Part print with two shaded views. Sizes in mm from the minimum x, y, z corner. Round coordinates to 2 decimals unless told otherwise and drop trailing zeros. Loops run counter-clockwise (first coordinate to the right, second up) from the corner with the lowest first, then second, coordinate; pieces in that order, holes last. Notation, with made-up numbers: M -6,-30.5 L 52,-30.5 A23 cw 52,-1.5 Z; hole C 66.25,11 d6. An arc over 180 degrees is marked long. Use a Markdown table: item, result. Add a question column.
Item 1: Wall check: L1, parallel to Z at x = 31, y = 95; L2, parallel to Y at x = 50, z = 13.25; L3, parallel to Z at x = 79, y = 85. Give the ranges that are in metal, low to high. Write a range as from..to.
Item 2: Pin check, flat tips, straight feed: P1, Ø10, axis at x = 58, z = 5.5, coming from the -Y side; P2, Ø1.5, axis at y = 71.5, z = 8, coming from the -X side; P3, Ø1.6, axis at x = 50, z = 11.5, coming from the -Y side. Stop position of each tip, or through.
Item 3: Saw through at A-A on y = 50. Write the cut outline in (x, z), then the cut area to 3 significant figures.
Item 4: Saw through at B-B on z = 8. Write the cut outline in (x, y), then the cut area to 3 significant figures.
Item 5: Two-plate mould, pull along Z, no slides. Class the marked faces 1, 2, 3 and 4: +Z half, -Z half, draft (parallel to the pull), parting line (faces both ways), or undercut.
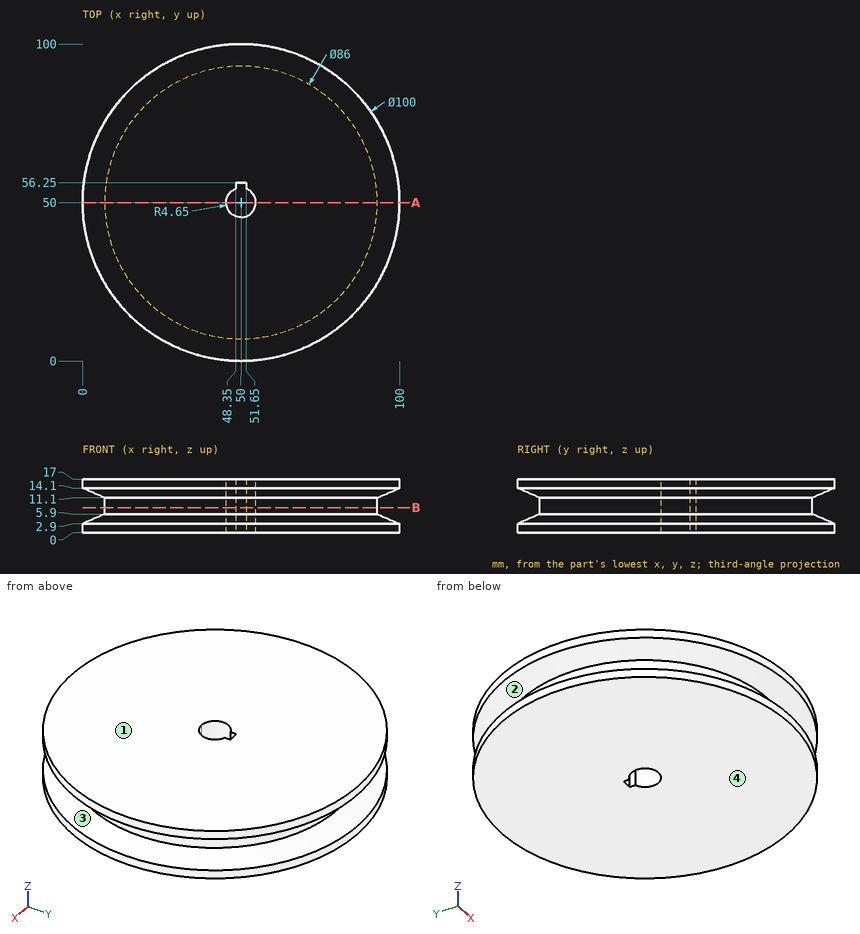
Entries:
| question | item | result |
|---|---|---|
| 1 | L1 | 0..3.39, 13.61..17 |
| 1 | L2 | 1.98..45.35, 56.25..98.02 |
| 1 | L3 | 0..4.85, 12.15..17 |
| 2 | P1 | y = 0.14 |
| 2 | P2 | x = 12.34 |
| 2 | P3 | y = 4.2 |
| 3 | outline | M 0,0 L 45.35,0 L 45.35,17 L 0,17 L 0,14.1 L 7,11.1 L 7,5.9 L 0,2.9 Z; M 54.65,0 L 100,0 L 100,2.9 L 93,5.9 L 93,11.1 L 100,14.1 L 100,17 L 54.65,17 Z |
| 3 | area | 1,430 mm2 |
| 4 | outline | C 50,50 d86; hole M 48.35,54.35 A4.65 ccw long 51.65,54.35 L 51.65,56.25 L 48.35,56.25 Z |
| 4 | area | 5,740 mm2 |
| 5 | face 1 | +Z half |
| 5 | face 2 | undercut |
| 5 | face 3 | undercut |
| 5 | face 4 | -Z half |
